For this review, take the finished solid that the model builds, in its own axes (mm). A direction names the side the tool comes from. Coordinates: 2 decimals unless noted, no trailing zeros. Loops run counter-clockwise (first coordinate to the right, second up) from the corner with the lowest first, then second, coordinate; pieces in that order, holes last. Notation, with made-up numbers: (42.25, 83) -> (92.25, 83) arc R32 cw to (92.25, 121) -> close; hole circle Ø8 at (-37, -4.5). An arc over 180 degrees is marked (long way). Use a Markdown table: item, result.
from build123d import *

# Parameters (mm, degrees)
IZIM1_R                     = 30
IZIM1_R_2                   = 10
Y_KSEKLIK_EKSTR_ZYON2_DEPTH = 25
IZIM1_4_R                   = 10
Y_KSEKLIK_EKSTR_ZYON3_DEPTH = 35
Y_KSEKLIK_EKSTR_ZYON4_START = -125
IZIM1_5_R                   = 30
IZIM1_5_R_2                 = 10
Y_KSEKLIK_EKSTR_ZYON4_DEPTH = 125
IZIM3_W                     = 54.543560574
IZIM3_H                     = 25
KES_EKSTR_ZYON1_DEPTH       = 115
KES_EKSTR_ZYON2_DEPTH       = 100
IZIM5_R                     = 4
KES_EKSTR_ZYON3_DEPTH       = 100
KES_EKSTR_ZYON4_DEPTH       = 5
KES_EKSTR_ZYON5_DEPTH       = 35.716373532
L_EK1_SCALE                 = 0.3


with BuildPart() as part:
    # Çizim1 → Yükseklik-Ekstrüzyon2 (new body)
    # profile 1 of 2: a face of its own
    with BuildSketch(Plane.XY):
        Circle(IZIM1_R)
        Circle(IZIM1_R_2, mode=Mode.SUBTRACT)
    # profile 2 of 2: a face of its own
    with BuildSketch(Plane.XY):
        Circle(IZIM1_R_2)
    extrude(amount=Y_KSEKLIK_EKSTR_ZYON2_DEPTH)

    # Çizim1<4> → Yükseklik-Ekstrüzyon3 (add)
    with BuildSketch(Plane.XY):
        Circle(IZIM1_4_R)
    extrude(amount=Y_KSEKLIK_EKSTR_ZYON3_DEPTH)

    # Çizim1<5> → Yükseklik-Ekstrüzyon4 (add)
    # profile 1 of 2: a face of its own
    with BuildSketch(Plane.XY.offset(Y_KSEKLIK_EKSTR_ZYON4_START)):
        Circle(IZIM1_5_R)
        Circle(IZIM1_5_R_2, mode=Mode.SUBTRACT)
    # profile 2 of 2: a face of its own
    with BuildSketch(Plane.XY.offset(Y_KSEKLIK_EKSTR_ZYON4_START)):
        Circle(IZIM1_5_R_2)
    extrude(amount=Y_KSEKLIK_EKSTR_ZYON4_DEPTH)

    # Çizim3 → Kes-Ekstrüzyon1 (cut)
    with BuildSketch(Plane(origin=(0, 0, -125), x_dir=(-1, 0, 0), z_dir=(0, 0, -1))):
        Rectangle(IZIM3_W, IZIM3_H)
        with BuildLine():
            Line((-27.271780287, -12.5), (-27.271780287, 12.5))
            ThreePointArc((-27.271780287, 12.5), (-30, 0), (-27.271780287, -12.5))
        make_face()
        with BuildLine():
            ThreePointArc((27.271780287, -12.5), (30, 0), (27.271780287, 12.5))
            Line((27.271780287, 12.5), (27.271780287, -12.5))
        make_face()
    extrude(amount=-KES_EKSTR_ZYON1_DEPTH, mode=Mode.SUBTRACT)

    # Çizim4 → Kes-Ekstrüzyon2 (cut)
    with BuildSketch(Plane(origin=(0, 0, -125), x_dir=(-1, 0, 0), z_dir=(0, 0, -1))):
        with BuildLine():
            Line((-19, 23.216373532), (19, 23.216373532))
            ThreePointArc((19, 23.216373532), (0, 30), (-19, 23.216373532))
        make_face()
        with BuildLine():
            Line((-19, -23.216373532), (19, -23.216373532))
            ThreePointArc((19, -23.216373532), (0, -30), (-19, -23.216373532))
        make_face()
    extrude(amount=-KES_EKSTR_ZYON2_DEPTH, mode=Mode.SUBTRACT)

    # Çizim5 → Kes-Ekstrüzyon3 (cut)
    with BuildSketch(Plane(origin=(0, 23.216373532, 0), x_dir=(1, 0, 0), z_dir=(0, 1, 0))):
        with Locations(Location((-8, 80, 0), (0, 0, 270))):
            Circle(IZIM5_R)
        with Locations(Location((8, 80, 0), (0, 0, 270))):
            Circle(IZIM5_R)
    extrude(amount=-KES_EKSTR_ZYON3_DEPTH, mode=Mode.SUBTRACT)

    # Çizim6 → Kes-Ekstrüzyon4 (cut)
    with BuildSketch(Plane(origin=(0, 23.216373532, 0), x_dir=(1, 0, 0), z_dir=(0, 1, 0))):
        with BuildLine():
            ThreePointArc((5, 106.843021333), (3.535533906, 110.378555239), (0, 111.843021333))
            Line((0, 111.843021333), (0, 101.843021333))
            ThreePointArc((0, 101.843021333), (3.535533906, 103.307487427), (5, 106.843021333))
        make_face()
        with BuildLine():
            Line((0, 101.843021333), (0, 111.843021333))
            ThreePointArc((0, 111.843021333), (-5, 106.843021333), (0, 101.843021333))
        make_face()
        with BuildLine():
            ThreePointArc((7.5, 106.843021333), (5.303300859, 112.146322192), (0, 114.343021333))
            Line((0, 114.343021333), (0, 111.843021333))
            ThreePointArc((0, 111.843021333), (3.535533906, 110.378555239), (5, 106.843021333))
            ThreePointArc((5, 106.843021333), (3.535533906, 103.307487427), (0, 101.843021333))
            Line((0, 101.843021333), (0, 99.343021333))
            ThreePointArc((0, 99.343021333), (5.303300859, 101.539720474), (7.5, 106.843021333))
        make_face()
        with BuildLine():
            Line((0, 111.843021333), (0, 114.343021333))
            ThreePointArc((0, 114.343021333), (-7.5, 106.843021333), (0, 99.343021333))
            Line((0, 99.343021333), (0, 101.843021333))
            ThreePointArc((0, 101.843021333), (-5, 106.843021333), (0, 111.843021333))
        make_face()
    kes_ekstr_zyon4 = extrude(amount=-KES_EKSTR_ZYON4_DEPTH, mode=Mode.SUBTRACT)

    # Çizim6<3> → Kes-Ekstrüzyon5 (cut)
    with BuildSketch(Plane(origin=(0, 23.216373532, 0), x_dir=(1, 0, 0), z_dir=(0, 1, 0))):
        with BuildLine():
            ThreePointArc((5, 106.843021333), (3.535533906, 110.378555239), (0, 111.843021333))
            Line((0, 111.843021333), (0, 101.843021333))
            ThreePointArc((0, 101.843021333), (3.535533906, 103.307487427), (5, 106.843021333))
        make_face()
        with BuildLine():
            Line((0, 101.843021333), (0, 111.843021333))
            ThreePointArc((0, 111.843021333), (-5, 106.843021333), (0, 101.843021333))
        make_face()
    kes_ekstr_zyon5 = extrude(amount=-KES_EKSTR_ZYON5_DEPTH, mode=Mode.SUBTRACT)

    # Aynalama1: Kes-Ekstrüzyon4, Kes-Ekstrüzyon5 across plane
    add(kes_ekstr_zyon4.mirror(Plane.ZX), mode=Mode.SUBTRACT)
    add(kes_ekstr_zyon5.mirror(Plane.ZX), mode=Mode.SUBTRACT)


with BuildPart() as part_1:
    # Ölçek1: scaled about (0, 0, -30.54358769)
    add(part.part.scale(L_EK1_SCALE).moved(Location((0, 0, -21.380511383))))


solid = part_1.part
(1) Take a section at B-B on y = 1.25. Write out the cut boundary in (x, z).
Found:
| item | result |
|---|---|
| outline | (-8.91, -24.38) -> (8.91, -24.38) -> (8.91, -13.88) -> (2.73, -13.88) -> (2.73, -10.88) -> (-2.73, -10.88) -> (-2.73, -13.88) -> (-8.91, -13.88) -> close |
(2) For faces 5 (the face through (0, -4, -13.881)), 6 (the face through (0, -3.75, -42)), 7 (the face through (0, 6.965, -44)), 8 (the face through (0, -6.965, -44)), list the 3-axis set-ups (+Z, -Z, +X, -X, +Y, -Y) from which the entire face can be reached by the end or side of a thin tool; tool diameter is ignored.
Found:
| item | result |
|---|---|
| face 5 | +Z |
| face 6 | -Z, +X, -X |
| face 7 | -Z, +X, -X, +Y |
| face 8 | -Z, +X, -X, -Y |
(3) Take a section at A-A on z = -31. Write out the cut boundary in (x, y), plus the area to 3 significant figures.
Found:
| item | result |
|---|---|
| outline | (-8.18, -3.75) arc R9 ccw to (-5.7, -6.96) -> (5.7, -6.96) arc R9 ccw to (8.18, -3.75) -> close; (-8.18, 3.75) -> (8.18, 3.75) arc R9 ccw to (5.7, 6.96) -> (-5.7, 6.96) arc R9 ccw to start |
| area | 91.8 mm^2 |
(4) For pin 1 Ø1 at (x, z) = (5, -31.5) entering from -Y; pin 2 Ø1 at (x, y) = (1, -7.5) entering from -Z; pin 3 Ø1 at (x, z) = (1, -51.5) entering from +Y; pin 4 Ø10 at (x, y) = (-4, 0.5) entering from -Z, all flat-tipped, find the tip position at first contact; note any pin that passes through.
Found:
| item | result |
|---|---|
| pin 1 | stops at y = -6.96 |
| pin 2 | stops at z = -28.88 |
| pin 3 | stops at y = 6.96 |
| pin 4 | stops at z = -58.88 |
(5) For line 1 along Y through (x, z) = (-1, -34); line 2 along Z through (x, y) = (6.5, -0.5); line 3 along Y through (x, z) = (-7.75, -45.5), list the stretches that pass through material, from the lowest coordinate up.
Found:
| item | result |
|---|---|
| line 1 | y = -6.96 to -3.75, 3.75 to 6.96 |
| line 2 | z = -24.38 to -13.88 |
| line 3 | y = -4.58 to -3.75, 3.75 to 4.58 |
(6) Take a section at C-C on x = -5.25. Write out the cut boundary in (y, z), plus the area to 3 significant figures.
Found:
| item | result |
|---|---|
| outline | (-7.31, -28.88) -> (-6.96, -28.88) -> (-6.96, -58.88) -> (-3.75, -58.88) -> (-3.75, -24.38) -> (3.75, -24.38) -> (3.75, -58.88) -> (6.96, -58.88) -> (6.96, -28.88) -> (7.31, -28.88) -> (7.31, -13.88) -> (-7.31, -13.88) -> close |
| area | 378 mm^2 |
(7) Take a section at D-D on z = -20.5. Write out the cut boundary in (x, y).
Found:
| item | result |
|---|---|
| outline | circle Ø18 at (0, 0) |
(8) Mouldability with a two-part tool opening along Z and no side actions: class faces 1 (the face through (-1, 5.465, -52)), 2 (the face through (-6.633, 6.083, -26.696)), 3 (the face through (-1, -5.465, -52)), 4 (the face through (0, -8, -28.881)) as pulls with the +Z half, pulls with the -Z half, needs draft (parallel to the pull), parting line crosses it, or undercut.
Found:
| item | result |
|---|---|
| face 1 | undercut |
| face 2 | needs draft |
| face 3 | undercut |
| face 4 | pulls with the -Z half |
